```python
from build123d import *

# Parameters (mm, degrees)
F1_R     = 2.032
F2_DEPTH = 5.842


with BuildPart() as f2:
    # F1 (on face) → F2 (new body)
    with BuildSketch(Plane.XY):
        with BuildLine():
            Line((254, -20.800026), (135.382, 0))
            ThreePointArc((135.382, 0), (113.548513, -73.722595), (55.090365, -123.666235))
            Line((55.090365, -123.666235), (32.373808, -135.382))
            Line((32.373808, -135.382), (253.931671, -135.382))
            Line((253.931671, -135.382), (254, -135.382))
            Line((254, -135.382), (254, -20.800026))
        make_face()
        with Locations((129.191592, -107.723273)):
            Circle(F1_R, mode=Mode.SUBTRACT)
        with Locations((148.749592, -107.723273)):
            Circle(F1_R, mode=Mode.SUBTRACT)
        with Locations((168.307592, -107.723273)):
            Circle(F1_R, mode=Mode.SUBTRACT)
        with Locations((187.865592, -107.723273)):
            Circle(F1_R, mode=Mode.SUBTRACT)
        with Locations((207.423592, -107.723273)):
            Circle(F1_R, mode=Mode.SUBTRACT)
        with Locations((226.981592, -107.723273)):
            Circle(F1_R, mode=Mode.SUBTRACT)
        with Locations((246.532425, -107.723273)):
            Circle(F1_R, mode=Mode.SUBTRACT)
    extrude(amount=F2_DEPTH)


solid = f2.part
```
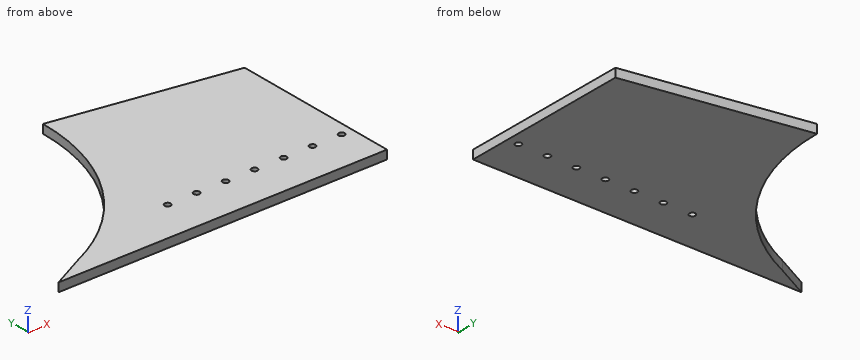
For this review, take the finished solid that the model builds, in its own axes (mm). Round coordinates to 2 decimals unless told otherwise and drop trailing zeros. Order: outer loops, then holes, each group sorted by start corner. A loop starts at its lowest first (then second) coordinate and runs counter-clockwise, first axis right, second up.
Q1. We need section C-C, the plane x = 222. Give the boundary of the cut face in (y, z), plus the area to 3 significant figures.
Findings below:
outline: (-135.38, 0) - (-15.19, 0) - (-15.19, 5.84) - (-135.38, 5.84) - close
area: 702 mm2
Q2. Wall thickness on line 1 (Y direction, x = 226.5, z = 1); line 2 (X direction, y = -66, z = 0.85); line 3 (Y direction, x = 158, z = 5.1): over which ranges is each line inside the solid? List them lowest first.
Findings below:
line 1: y = -135.38 to -109.7, -105.75 to -15.98
line 2: x = 118.2 to 254
line 3: y = -135.38 to -3.97
Q3. We need section A-A, the plane z = 4.6. Give the boundary of the cut face in (x, y), plus the area to 3 significant figures.
Findings below:
outline: (32.37, -135.38) - (254, -135.38) - (254, -20.8) - (135.38, 0) arc R135.38 cw to (55.09, -123.67) - close; hole circle Ø4.06 at (129.19, -107.72); hole circle Ø4.06 at (148.75, -107.72); hole circle Ø4.06 at (168.31, -107.72); hole circle Ø4.06 at (187.87, -107.72); hole circle Ø4.06 at (207.42, -107.72); hole circle Ø4.06 at (226.98, -107.72); hole circle Ø4.06 at (246.53, -107.72)
area: 18,600 mm2
Q4. We need section B-B, the plane y = -61.5. Give the boundary of the cut face in (x, z), plus the area to 3 significant figures.
Findings below:
outline: (120.61, 0) - (254, 0) - (254, 5.84) - (120.61, 5.84) - close
area: 779 mm2
